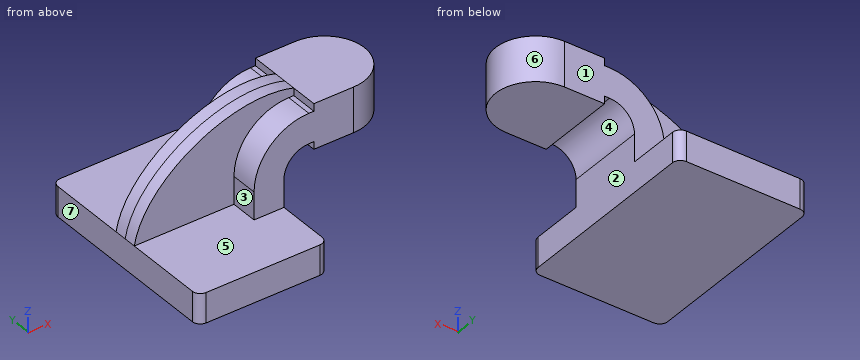
from build123d import *

# Parameters (mm, degrees)
F1_DEPTH = 63.5
F2_DEPTH = 25.4
F3_DEPTH = 7.9375
F0_W     = 25.4
F0_H     = 28.575
F5_R     = 5.08


with BuildPart() as f1:
    # F0 (on Front) → F1 (new body, symmetric)
    with BuildSketch(Plane.XZ):
        Polygon((-41.275, -9.525), (41.275, -9.525), (41.275, 9.525), (22.225, 9.525), (-41.275, 9.525), align=None)
    extrude(amount=F1_DEPTH, both=True)

    # F0 (on Front) → F2 (join, symmetric)
    with BuildSketch(Plane.XZ):
        with BuildLine():
            Line((22.225, 9.525), (41.275, 9.525))
            Line((41.275, 9.525), (41.275, 27.0002))
            ThreePointArc((41.275, 27.0002), (45.92468, 38.22552), (57.15, 42.8752))
            Line((57.15, 42.8752), (60.325, 42.8752))
            Line((60.325, 42.8752), (60.325, 61.9252))
            Line((60.325, 61.9252), (57.15, 61.9252))
            ThreePointArc((57.15, 61.9252), (32.454296, 51.695904), (22.225, 27.0002))
            Line((22.225, 27.0002), (22.225, 9.525))
        make_face()
        Polygon((85.725, 66.675), (60.325, 66.675), (60.325, 61.9252), (60.325, 42.8752), (60.325, 38.1), (85.725, 38.1), align=None)
    extrude(amount=F2_DEPTH, both=True)

    # F0 (on Front) → F3 (join, symmetric)
    with BuildSketch(Plane.XZ):
        with BuildLine():
            add(Edge.make_bspline(
                [(-41.275, 9.525), (-34.780891, 47.233644), (21.640048, 78.397568), (60.325, 66.675)],
                knots=[0, 0, 0, 0, 116.570504, 116.570504, 116.570504, 116.570504], degree=3))
            Line((-41.275, 9.525), (22.225, 9.525))
            Line((22.225, 9.525), (22.225, 27.0002))
            ThreePointArc((22.225, 27.0002), (32.454296, 51.695904), (57.15, 61.9252))
            Line((57.15, 61.9252), (60.325, 61.9252))
            Line((60.325, 61.9252), (60.325, 66.675))
        make_face()
    extrude(amount=F3_DEPTH, both=True)

    # F0 (on Front) → F4 (revolve)
    with BuildSketch(Plane.XZ):
        with Locations((98.425, 52.3875)):
            Rectangle(F0_W, F0_H)
    revolve(axis=Axis((85.725, 0, 52.3875), (0, 0, 1)))

    # F5
    f5_edges = [f1.edges().sort_by_distance(p)[0] for p in [
        (41.275, -63.5, 0),
        (-41.275, -63.5, 0),
        (-41.275, 63.5, 0),
        (41.275, 63.5, 0),
    ]]
    fillet(f5_edges, radius=F5_R)


solid = f1.part
Could you check a few things on this model? Use its own coordinates, in mm. Face numbers are marked on the shaded views. A direction names the side the tool comes from. Coordinates: 2 decimals unless noted, no trailing zeros. Loops run counter-clockwise (first coordinate to the right, second up) from the corner with the lowest first, then second, coordinate; pieces in that order, holes last.
1. I need wall thicknesses on L1, parallel to X at y = -51, z = -2 (3 decimals); L2, parallel to Z at x = 66, y = 15 (3 decimals); L3, parallel to Z at x = 24, y = -27.5 (3 decimals). Which ranges of each line are inside material? Lowest first, please.
2. For the marked faces 1, 2 and 3, which set-ups out of +Z, -Z, +X, -X, +Y, -Y let a thin tool reach every point of the face, with its end or its side?
3. For P1, Ø3.5, axis at x = 59, y = 2, coming from the -Z side; P2, Ø8.5, axis at y = 19, z = 14, coming from the -X side (3 decimals); P3, Ø2.5, axis at y = -19, z = 64.5, coming from the -X side (3 decimals); P4, Ø5, axis at x = 20, z = 11.5, coming from the +Y side, each with a flat end and sliding along its axis, tell me the tip position at first contact or that it passes through.
4. Imagine slicing it at B-B (x = 84). Please give me the cut outline in (y, z) (3 decimals).
5. Imagine slicing it at A-A (y = -37). Please give me the cut outline in (x, z) (3 decimals), and give its area (3 significant figures).
6. We'd pull the mould along X, two halves only. Please class the marked faces 4, 5, 6 and 7: released by +X, released by -X, zero draft, split by the parting line, or undercut.
Computed values:
1. L1: x = -41.275 to 41.275
1. L2: z = 38.1 to 66.675
1. L3: z = -9.525 to 9.525
2. face 1: +Z, +X, -X, +Y
2. face 2: -Z, +X, +Y, -Y
2. face 3: +Z, -X, -Y
3. P1: stops at z = 38.1
3. P2: stops at x = 22.225
3. P3: stops at x = 60.325
3. P4: stops at y = 63.5
4. outline: (-25.4, 38.1) - (25.4, 38.1) - (25.4, 66.675) - (-25.4, 66.675) - close
5. outline: (-41.275, -9.525) - (41.275, -9.525) - (41.275, 9.525) - (-41.275, 9.525) - close
5. area: 1,570 mm2
6. face 4: undercut
6. face 5: zero draft
6. face 6: released by +X
6. face 7: released by -X
